```python
from build123d import *

# Parameters (mm, degrees)
EXTRUDE_1_OUTLINE_R      = 30
EXTRUDE_1_OUTLINE_R_2    = 1.5
EXTRUDE_1_OUTLINE_R_3    = 26
EXTRUDE_1_DEPTH          = 8
CUT_EXTRUDE_1_DEPTH      = 44.17406629
CUT_EXTRUDE_1_DEPTH_BACK = 44.17406629
CUT_EXTRUDE_2_DEPTH      = 44.174066447
CUT_EXTRUDE_2_DEPTH_BACK = 44.174066447
SKETCH_5_R               = 1.9


# Read off the part's stored shape, not the designer's step: 凸台-拉伸1
with BuildPart() as part:
    # 凸台-拉伸1 outline → 凸台-拉伸1 (new body)
    with BuildSketch(Plane(origin=(0, 0, 0), x_dir=(1, 0, 0), z_dir=(0, 1, 0))):
        Circle(EXTRUDE_1_OUTLINE_R)
        with Locations((-19.798989873, -19.798989873)):
            Circle(EXTRUDE_1_OUTLINE_R_2, mode=Mode.SUBTRACT)
        with Locations((0, -28)):
            Circle(EXTRUDE_1_OUTLINE_R_2, mode=Mode.SUBTRACT)
        with Locations((19.798989873, -19.798989873)):
            Circle(EXTRUDE_1_OUTLINE_R_2, mode=Mode.SUBTRACT)
        with Locations((-28, 0)):
            Circle(EXTRUDE_1_OUTLINE_R_2, mode=Mode.SUBTRACT)
        with Locations((-19.798989873, 19.798989873)):
            Circle(EXTRUDE_1_OUTLINE_R_2, mode=Mode.SUBTRACT)
        Circle(EXTRUDE_1_OUTLINE_R_3, mode=Mode.SUBTRACT)
        with Locations((28, 0)):
            Circle(EXTRUDE_1_OUTLINE_R_2, mode=Mode.SUBTRACT)
        with Locations((0, 28)):
            Circle(EXTRUDE_1_OUTLINE_R_2, mode=Mode.SUBTRACT)
        with Locations((19.798989873, 19.798989873)):
            Circle(EXTRUDE_1_OUTLINE_R_2, mode=Mode.SUBTRACT)
    extrude(amount=EXTRUDE_1_DEPTH)

    # 草图4 → 切除-拉伸1 (cut, two sides: drawn at the far end of the back side and taken through both)
    with BuildSketch(Plane(origin=(0, 0, 0), x_dir=(-0.38268343236509067, 0, -0.9238795325112864), z_dir=(0.9238795325112864, 0, -0.38268343236509067)).offset(-CUT_EXTRUDE_1_DEPTH_BACK)):
        with BuildLine():
            ThreePointArc((0, 5.9), (-1.9, 4), (0, 2.1))
            Line((0, 2.1), (0, 5.9))
        make_face()
        with BuildLine():
            Line((0, 5.9), (0, 2.1))
            ThreePointArc((0, 2.1), (1.343502884, 2.656497116), (1.9, 4))
            ThreePointArc((1.9, 4), (1.343502884, 5.343502884), (0, 5.9))
        make_face()
    extrude(amount=CUT_EXTRUDE_1_DEPTH + CUT_EXTRUDE_1_DEPTH_BACK, mode=Mode.SUBTRACT)

    # 草图5 → 切除-拉伸2 (cut, two sides: drawn at the far end of the back side and taken through both)
    with BuildSketch(Plane(origin=(0, 0, 0), x_dir=(0.9238795325112864, 0, -0.3826834323650906), z_dir=(0.3826834323650906, 0, 0.9238795325112864)).offset(-CUT_EXTRUDE_2_DEPTH_BACK)):
        with Locations((0, 4)):
            Circle(SKETCH_5_R)
    extrude(amount=CUT_EXTRUDE_2_DEPTH + CUT_EXTRUDE_2_DEPTH_BACK, mode=Mode.SUBTRACT)


solid = part.part
```
Check sheet for the modelled part. Datum: model origin and axes. Units: mm. Give positions to 0.01 mm unless a question says otherwise; leave off trailing zeros. Write each loop counter-clockwise with the first axis right and the second up, starting at its lowest first coordinate (ties: lowest second). Pieces come first, ordered by that corner, then holes. Notation, with made-up numbers: (-30.75, -8.5) - (26.25, -8.5) arc R21 ccw to (26.25, 25.5) - close; hole circle Ø8 at (54, -22.75). An arc over 180 degrees is marked (long way). Answer as a JSON object with one key per item and string values. Group by question number.
1) Sectioned sample at A-A (z = 0). Record the cut outline in (x, y).
2) Depth check by flat-ended pin: P1, Ø1.5, axis at x = -7, y = 6.5, coming from the -Z side; P2, Ø3.5, axis at x = -28, z = 0, coming from the +Y side; P3, Ø1, axis at x = -1, y = 2.5, coming from the -Z side; P4, Ø2, axis at y = 2, z = -10, coming from the -X side. Enter the tip coordinate at first touch or a pass-through.
3) Sectioned sample at C-C (y = 3). Give the number of separate pieces and of enclosed holes in the cut face, then the cut area to 3 significant figures.
4) Sectioned sample at D-D (z = -17). Record the cut outline in (x, y).
5) Thickness scan on probe 1 along X at (y, z) = (3.75, 0); probe 2 along X at (y, z) = (5.25, -20); probe 3 along Z at (x, y) = (-17, 1.5). Record the ranges inside material, lowest first. Write a range as from..to.
6) Sectioned sample at B-B (x = 0). Record the cut outline in (y, z), then the cut area to 3 significant figures.
7) Release check for a two-part mould opening along Z. For faces 1 (the face through (-13.5, 0, -22.4)), 2 (the face through (-29.97, 3.94, -1.32)), 3 (the face through (-12.01, 5.28, -25.33)) record: pulls with the +Z half, pulls with the -Z half, needs draft (parallel to the pull), parting line crosses it, or undercut.
Geometry results:
{
 "1": {"outline": "(-30, 0) - (-29.5, 0) - (-29.5, 8) - (-30, 8) - close; (-26.5, 0) - (-26, 0) - (-26, 8) - (-26.5, 8) - close; (26, 0) - (26.5, 0) - (26.5, 8) - (26, 8) - close; (29.5, 0) - (30, 0) - (30, 8) - (29.5, 8) - close"},
 "2": {"P1": "stops at z = -29.34", "P2": "stops at y = 8", "P3": "stops at z = -30", "P4": "stops at x = -28.62"},
 "3": {"separate pieces": "4", "enclosed holes": "8", "area": "595 mm^2"},
 "4": {"outline": "(-24.72, 0) - (-19.67, 0) - (-19.67, 8) - (-24.72, 8) - close; (19.67, 0) - (24.72, 0) - (24.72, 8) - (19.67, 8) - close"},
 "5": {"probe 1": "x = -30..-29.5, -26.5..-26, 26..26.5, 29.5..30", "probe 2": "x = -22.36..-21.29, -18.31..-16.61, 16.61..18.31, 21.29..22.36", "probe 3": "z = -24.72..-19.67, 19.67..24.72"},
 "6": {"outline": "(0, -30) - (8, -30) - (8, -29.5) - (0, -29.5) - close; (0, -26.5) - (8, -26.5) - (8, -26) - (0, -26) - close; (0, 26) - (8, 26) - (8, 26.5) - (0, 26.5) - close; (0, 29.5) - (8, 29.5) - (8, 30) - (0, 30) - close", "area": "16.0 mm^2"},
 "7": {"face 1": "needs draft", "face 2": "parting line crosses it", "face 3": "undercut"}
}
